```python
from build123d import *

# Parameters (mm, degrees)
EXTRUDE_1_DEPTH        = 25
CUT_EXTRUDE_1_DEPTH    = 53.585134746
EXTRUDE_2_DEPTH        = 4
SKETCH_4_R             = 3.5
SKETCH_4_R_2           = 1.7
SKETCH_4_R_3           = 2.3
CUT_EXTRUDE_2_DEPTH    = 55.600333298
SKETCH_5_R             = 50
CUT_EXTRUDE_3_DEPTH    = 4
HOLE_WIZARD_M3_1_D     = 2.5
HOLE_WIZARD_M3_1_DEPTH = 11.5
HOLE_WIZARD_M3_1_TIP   = 0.751075774


with BuildPart() as part:
    # 草图1 → 凸台-拉伸1 (new body)
    with BuildSketch(Plane.XY):
        with BuildLine():
            Line((15.936762996, 30.229618981), (13.50337588, 31.175538906))
            ThreePointArc((13.50337588, 31.175538906), (11.545587701, 31.113280948), (10.233613318, 29.658793469))
            ThreePointArc((10.233613318, 29.658793469), (6.285609854, 24.369935979), (0, 22.357511157))
            ThreePointArc((0, 22.357511157), (-6.541634269, 25.176328334), (-8.985563862, 31.867062025))
            ThreePointArc((-8.985563862, 31.867062025), (-9.328351981, 32.569720668), (-10.106575389, 32.644561759))
            Line((-10.106575389, 32.644561759), (-12.496106314, 31.592763621))
            ThreePointArc((-12.496106314, 31.592763621), (-13.836448588, 30.1643753), (-13.73567661, 28.208191357))
            ThreePointArc((-13.73567661, 28.208191357), (-12.787549636, 21.67674434), (-15.80914775, 15.80914775))
            ThreePointArc((-15.80914775, 15.80914775), (-22.427986442, 13.176718539), (-28.887168794, 16.179662515))
            ThreePointArc((-28.887168794, 16.179662515), (-29.626411288, 16.434129403), (-30.229618981, 15.936762996))
            Line((-30.229618981, 15.936762996), (-31.175538906, 13.50337588))
            ThreePointArc((-31.175538906, 13.50337588), (-31.113280948, 11.545587701), (-29.658793469, 10.233613318))
            ThreePointArc((-29.658793469, 10.233613318), (-24.369935979, 6.285609854), (-22.357511157, 0))
            ThreePointArc((-22.357511157, 0), (-25.176328334, -6.541634269), (-31.867062025, -8.985563862))
            ThreePointArc((-31.867062025, -8.985563862), (-32.569720668, -9.328351981), (-32.644561759, -10.106575389))
            Line((-32.644561759, -10.106575389), (-31.592763621, -12.496106314))
            ThreePointArc((-31.592763621, -12.496106314), (-30.1643753, -13.836448588), (-28.208191357, -13.73567661))
            ThreePointArc((-28.208191357, -13.73567661), (-21.67674434, -12.787549636), (-15.80914775, -15.80914775))
            ThreePointArc((-15.80914775, -15.80914775), (-13.176718539, -22.427986442), (-16.179662515, -28.887168794))
            ThreePointArc((-16.179662515, -28.887168794), (-16.434129403, -29.626411288), (-15.936762996, -30.229618981))
            Line((-15.936762996, -30.229618981), (-13.50337588, -31.175538906))
            ThreePointArc((-13.50337588, -31.175538906), (-11.545587701, -31.113280948), (-10.233613318, -29.658793469))
            ThreePointArc((-10.233613318, -29.658793469), (-6.285609854, -24.369935979), (0, -22.357511157))
            ThreePointArc((0, -22.357511157), (6.541634269, -25.176328334), (8.985563862, -31.867062025))
            ThreePointArc((8.985563862, -31.867062025), (9.328351981, -32.569720668), (10.106575389, -32.644561759))
            Line((10.106575389, -32.644561759), (12.496106314, -31.592763621))
            ThreePointArc((12.496106314, -31.592763621), (13.836448588, -30.1643753), (13.73567661, -28.208191357))
            ThreePointArc((13.73567661, -28.208191357), (12.787549636, -21.67674434), (15.80914775, -15.80914775))
            ThreePointArc((15.80914775, -15.80914775), (22.427986442, -13.176718539), (28.887168794, -16.179662515))
            ThreePointArc((28.887168794, -16.179662515), (29.626411288, -16.434129403), (30.229618981, -15.936762996))
            Line((30.229618981, -15.936762996), (31.175538906, -13.50337588))
            ThreePointArc((31.175538906, -13.50337588), (31.113280948, -11.545587701), (29.658793469, -10.233613318))
            ThreePointArc((29.658793469, -10.233613318), (24.369935979, -6.285609854), (22.357511157, 0))
            ThreePointArc((22.357511157, 0), (25.176328334, 6.541634269), (31.867062025, 8.985563862))
            ThreePointArc((31.867062025, 8.985563862), (32.569720668, 9.328351981), (32.644561759, 10.106575389))
            Line((32.644561759, 10.106575389), (31.592763621, 12.496106314))
            ThreePointArc((31.592763621, 12.496106314), (30.1643753, 13.836448588), (28.208191357, 13.73567661))
            ThreePointArc((28.208191357, 13.73567661), (21.67674434, 12.787549636), (15.80914775, 15.80914775))
            ThreePointArc((15.80914775, 15.80914775), (13.176718539, 22.427986442), (16.179662515, 28.887168794))
            ThreePointArc((16.179662515, 28.887168794), (16.434129403, 29.626411288), (15.936762996, 30.229618981))
        make_face()
    extrude(amount=EXTRUDE_1_DEPTH)

    # 草图2 → 切除-拉伸1 (cut, through all)
    with BuildSketch(Plane(origin=(0, 0, 0), x_dir=(-1, 0, 0), z_dir=(0, 0, -1))):
        with BuildLine():
            ThreePointArc((20.357511157, 0), (21.09666185, -3.964211334), (23.214778703, -7.395668204))
            ThreePointArc((23.214778703, -7.395668204), (23.607260601, -9.441727167), (21.96737362, -10.726705772))
            ThreePointArc((21.96737362, -10.726705772), (17.87170053, -11.922005636), (14.394934187, -14.394934187))
            ThreePointArc((14.394934187, -14.394934187), (12.114471938, -17.720713371), (11.185800306, -21.644854583))
            ThreePointArc((11.185800306, -21.644854583), (10.01654475, -23.369163362), (7.948352461, -23.118205243))
            ThreePointArc((7.948352461, -23.118205243), (4.207069606, -21.067331667), (0, -20.357511157))
            ThreePointArc((0, -20.357511157), (-3.964211334, -21.09666185), (-7.395668204, -23.214778703))
            ThreePointArc((-7.395668204, -23.214778703), (-9.441727167, -23.607260601), (-10.726705772, -21.96737362))
            ThreePointArc((-10.726705772, -21.96737362), (-11.922005636, -17.87170053), (-14.394934187, -14.394934187))
            ThreePointArc((-14.394934187, -14.394934187), (-17.720713371, -12.114471938), (-21.644854583, -11.185800306))
            ThreePointArc((-21.644854583, -11.185800306), (-23.369163362, -10.01654475), (-23.118205243, -7.948352461))
            ThreePointArc((-23.118205243, -7.948352461), (-21.067331667, -4.207069606), (-20.357511157, 0))
            ThreePointArc((-20.357511157, 0), (-21.09666185, 3.964211334), (-23.214778703, 7.395668204))
            ThreePointArc((-23.214778703, 7.395668204), (-23.607260601, 9.441727167), (-21.96737362, 10.726705772))
            ThreePointArc((-21.96737362, 10.726705772), (-17.87170053, 11.922005636), (-14.394934187, 14.394934187))
            ThreePointArc((-14.394934187, 14.394934187), (-12.114471938, 17.720713371), (-11.185800306, 21.644854583))
            ThreePointArc((-11.185800306, 21.644854583), (-10.01654475, 23.369163362), (-7.948352461, 23.118205243))
            ThreePointArc((-7.948352461, 23.118205243), (-4.207069606, 21.067331667), (0, 20.357511157))
            ThreePointArc((0, 20.357511157), (3.964211334, 21.09666185), (7.395668204, 23.214778703))
            ThreePointArc((7.395668204, 23.214778703), (9.441727167, 23.607260601), (10.726705772, 21.96737362))
            ThreePointArc((10.726705772, 21.96737362), (11.922005636, 17.87170053), (14.394934187, 14.394934187))
            ThreePointArc((14.394934187, 14.394934187), (17.720713371, 12.114471938), (21.644854583, 11.185800306))
            ThreePointArc((21.644854583, 11.185800306), (23.369163362, 10.01654475), (23.118205243, 7.948352461))
            ThreePointArc((23.118205243, 7.948352461), (21.067331667, 4.207069606), (20.357511157, 0))
        make_face()
    extrude(amount=-CUT_EXTRUDE_1_DEPTH, mode=Mode.SUBTRACT)

    # 草图3 → 凸台-拉伸2 (add)
    with BuildSketch(Plane.XY.offset(25)):
        with BuildLine():
            Line((15.936762996, 30.229618981), (13.50337588, 31.175538906))
            ThreePointArc((13.50337588, 31.175538906), (11.545587701, 31.113280948), (10.233613318, 29.658793469))
            ThreePointArc((10.233613318, 29.658793469), (6.285609854, 24.369935979), (0, 22.357511157))
            ThreePointArc((0, 22.357511157), (-6.541634269, 25.176328334), (-8.985563862, 31.867062025))
            ThreePointArc((-8.985563862, 31.867062025), (-9.328351981, 32.569720668), (-10.106575389, 32.644561759))
            Line((-10.106575389, 32.644561759), (-12.496106314, 31.592763621))
            ThreePointArc((-12.496106314, 31.592763621), (-13.836448588, 30.1643753), (-13.73567661, 28.208191357))
            ThreePointArc((-13.73567661, 28.208191357), (-12.787549636, 21.67674434), (-15.80914775, 15.80914775))
            ThreePointArc((-15.80914775, 15.80914775), (-22.427986442, 13.176718539), (-28.887168794, 16.179662515))
            ThreePointArc((-28.887168794, 16.179662515), (-29.626411288, 16.434129403), (-30.229618981, 15.936762996))
            Line((-30.229618981, 15.936762996), (-31.175538906, 13.50337588))
            ThreePointArc((-31.175538906, 13.50337588), (-31.113280948, 11.545587701), (-29.658793469, 10.233613318))
            ThreePointArc((-29.658793469, 10.233613318), (-24.369935979, 6.285609854), (-22.357511157, 0))
            ThreePointArc((-22.357511157, 0), (-25.176328334, -6.541634269), (-31.867062025, -8.985563862))
            ThreePointArc((-31.867062025, -8.985563862), (-32.569720668, -9.328351981), (-32.644561759, -10.106575389))
            Line((-32.644561759, -10.106575389), (-31.592763621, -12.496106314))
            ThreePointArc((-31.592763621, -12.496106314), (-30.1643753, -13.836448588), (-28.208191357, -13.73567661))
            ThreePointArc((-28.208191357, -13.73567661), (-21.67674434, -12.787549636), (-15.80914775, -15.80914775))
            ThreePointArc((-15.80914775, -15.80914775), (-13.176718539, -22.427986442), (-16.179662515, -28.887168794))
            ThreePointArc((-16.179662515, -28.887168794), (-16.434129403, -29.626411288), (-15.936762996, -30.229618981))
            Line((-15.936762996, -30.229618981), (-13.50337588, -31.175538906))
            ThreePointArc((-13.50337588, -31.175538906), (-11.545587701, -31.113280948), (-10.233613318, -29.658793469))
            ThreePointArc((-10.233613318, -29.658793469), (-6.285609854, -24.369935979), (0, -22.357511157))
            ThreePointArc((0, -22.357511157), (6.541634269, -25.176328334), (8.985563862, -31.867062025))
            ThreePointArc((8.985563862, -31.867062025), (9.328351981, -32.569720668), (10.106575389, -32.644561759))
            Line((10.106575389, -32.644561759), (12.496106314, -31.592763621))
            ThreePointArc((12.496106314, -31.592763621), (13.836448588, -30.1643753), (13.73567661, -28.208191357))
            ThreePointArc((13.73567661, -28.208191357), (12.787549636, -21.67674434), (15.80914775, -15.80914775))
            ThreePointArc((15.80914775, -15.80914775), (22.427986442, -13.176718539), (28.887168794, -16.179662515))
            ThreePointArc((28.887168794, -16.179662515), (29.626411288, -16.434129403), (30.229618981, -15.936762996))
            Line((30.229618981, -15.936762996), (31.175538906, -13.50337588))
            ThreePointArc((31.175538906, -13.50337588), (31.113280948, -11.545587701), (29.658793469, -10.233613318))
            ThreePointArc((29.658793469, -10.233613318), (24.369935979, -6.285609854), (22.357511157, 0))
            ThreePointArc((22.357511157, 0), (25.176328334, 6.541634269), (31.867062025, 8.985563862))
            ThreePointArc((31.867062025, 8.985563862), (32.569720668, 9.328351981), (32.644561759, 10.106575389))
            Line((32.644561759, 10.106575389), (31.592763621, 12.496106314))
            ThreePointArc((31.592763621, 12.496106314), (30.1643753, 13.836448588), (28.208191357, 13.73567661))
            ThreePointArc((28.208191357, 13.73567661), (21.67674434, 12.787549636), (15.80914775, 15.80914775))
            ThreePointArc((15.80914775, 15.80914775), (13.176718539, 22.427986442), (16.179662515, 28.887168794))
            ThreePointArc((16.179662515, 28.887168794), (16.434129403, 29.626411288), (15.936762996, 30.229618981))
        make_face()
    extrude(amount=EXTRUDE_2_DEPTH)

    # 草图4 → 切除-拉伸2 (cut, through all)
    with BuildSketch(Plane.XY.offset(29)):
        Circle(SKETCH_4_R)
        with Locations((8, 0)):
            Circle(SKETCH_4_R_2)
        with Locations((0, -8)):
            Circle(SKETCH_4_R_2)
        with Locations((-8, 0)):
            Circle(SKETCH_4_R_2)
        with Locations((0, 8)):
            Circle(SKETCH_4_R_2)
        with Locations((-9.234972265, 17.740216664)):
            Circle(SKETCH_4_R_3)
        with Locations((17.740216664, 9.234972265)):
            Circle(SKETCH_4_R_3)
        with Locations((9.234972265, -17.740216664)):
            Circle(SKETCH_4_R_3)
        with Locations((-17.740216664, -9.234972265)):
            Circle(SKETCH_4_R_3)
    extrude(amount=-CUT_EXTRUDE_2_DEPTH, mode=Mode.SUBTRACT)

    # 草图5 → 切除-拉伸3 (cut)
    with BuildSketch(Plane.XY.offset(29)):
        Circle(SKETCH_5_R)
    extrude(amount=-CUT_EXTRUDE_3_DEPTH, mode=Mode.SUBTRACT)

    # M3 螺纹孔1
    with Locations(Plane.XY.offset(25)):
        with Locations((-10.95008804, 27.930191047), (12.006745981, 27.492508997), (27.930191047, 10.95008804), (27.492508997, -12.006745981), (10.95008804, -27.930191047), (-12.006745981, -27.492508997), (-27.930191047, -10.95008804), (-27.492508997, 12.006745981)):
            Hole(HOLE_WIZARD_M3_1_D / 2, depth=HOLE_WIZARD_M3_1_DEPTH)
            with Locations((0, 0, -(HOLE_WIZARD_M3_1_DEPTH + HOLE_WIZARD_M3_1_TIP / 2))):  # 118° drill point
                Cone(0, HOLE_WIZARD_M3_1_D / 2, HOLE_WIZARD_M3_1_TIP, mode=Mode.SUBTRACT)


solid = part.part
```
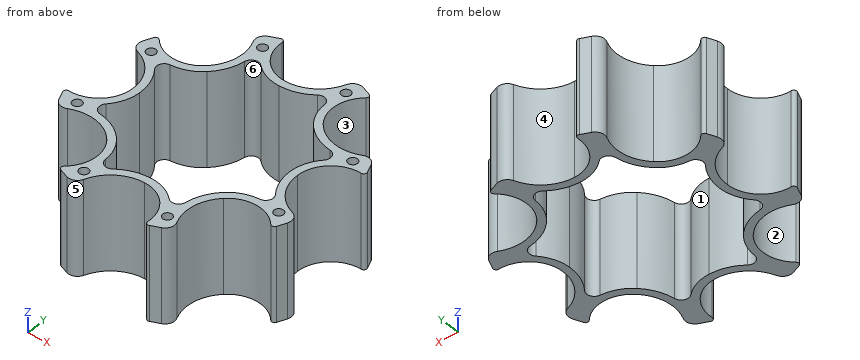
Work out the finished part from the listing and answer in its coordinate system (mm). Face numbers are marked on the shaded views. A direction names the side the tool comes from. Round coordinates to 2 decimals unless told otherwise and drop trailing zeros. Write each loop counter-clockwise with the first axis right and the second up, starting at its lowest first coordinate (ties: lowest second). Pieces come first, ordered by that corner, then holes.
1) Determine the mould class of the marked faces 1, 2 and 3 for opening direction X: pulls with the +X half, pulls with the -X half, needs draft (parallel to the pull), parting line crosses it, or undercut.
2) A cutting plane is placed at B-B on y = 3.5. Determine the outline of the cut face in (x, z).
3) Consider probe 1 along Y at (x, z) = (27.5, 17.5); probe 2 along Y at (x, z) = (10, 14.5); probe 3 along X at (y, z) = (15.5, 21.5). Determine where each line is inside the solid, lowest interval first.
4) Flat-ended cylindrical pins translate along their axes: P1, Ø5, axis at x = -20, z = 21, coming from the -Y side; P2, Ø4, axis at y = -1.5, z = 14, coming from the -X side; P3, Ø6, axis at x = 15.5, z = 21.5, coming from the +Y side. Find the tip coordinate at first contact, or state that the pin passes through.
5) Which of the six approach directions +Z, -Z, +X, -X, +Y, -Y give full straight-line access (tool end or side, diameter ignored) to the marked faces 4, 5 and 6?
6) A cutting plane is placed at A-A on x = -2.5. Determine the outline of the cut face in (y, z).
7) A cutting plane is placed at C-C on z = 21.5. Give the number of separate pieces and of enclosed holes in the cut face, and give its area (3 significant figures).
Entries:
1. face 1: undercut
1. face 2: pulls with the -X half
1. face 3: pulls with the +X half
2. outline: (-22.94, 0) - (-20.84, 0) - (-20.84, 25) - (-22.94, 25) - close; (20.93, 0) - (23.07, 0) - (23.07, 25) - (20.93, 25) - close
3. probe 1: y = -14.92 to -13.26, -10.76 to -9.21, 8.13 to 9.78, 12.12 to 13.42
3. probe 2: y = -32.68 to -28.74, -27.12 to -23.29, 23.38 to 29.04
3. probe 3: x = -30.4 to -28.21, -16.13 to -13.41, 13.43 to 16.13
4. P1: stops at y = -14.43
4. P2: stops at x = -23.07
4. P3: stops at y = 31.35
5. face 4: +Z, -Z, +Y
5. face 5: +Z, -Z, -Y
5. face 6: +Z, -Z
6. outline: (-22.65, 0) - (-20.6, 0) - (-20.6, 25) - (-22.65, 25) - close; (20.65, 0) - (22.71, 0) - (22.71, 25) - (20.65, 25) - close
7. separate pieces: 1
7. enclosed holes: 9
7. area: 597 mm2
